Could you check a few things on this model? Use its own coordinates, in mm. A direction names the side the tool comes from. Coordinates: 2 decimals unless noted, no trailing zeros. Write each loop counter-clockwise with the first axis right and the second up, starting at its lowest first coordinate (ties: lowest second). Pieces come first, ordered by that corner, then holes. Notation, with made-up numbers: M 89.25,-30 L 123.25,-30 A7 ccw 123.25,-19 Z; hole C 46,-17.75 d2. An arc over 180 degrees is marked long. Answer as CSV lines item,"result". Start each with the question number.
Item 1: On a 3-axis mill with a long thin cutter (end or side, diameter ignored), from which of +Z, -Z, +X, -X, +Y, -Y can I reach the whole of each face in a straight line? I mean faces 4 (the cylindrical face through (-15.07, 3.24, 10.32)), 5 (the flat face through (15, 4.5, 4)), 6 (the flat face through (-15, -4.5, 4)), 7 (the flat face through (15, -4.5, 4)). Say none if no direction works.
Item 2: I'm going to push flat-ended pins straight in: P1, Ø3, axis at x = 14.5, z = 3.5, coming from the +Y side; P2, Ø1.5, axis at y = 6.5, z = 8.5, coming from the +X side; P3, Ø6.5, axis at x = 16, z = 4, coming from the -Y side; P4, Ø2.5, axis at y = 0, z = 6.6, coming from the +X side. Where does each tip first touch, or does it pass through?
Item 3: Suppose I cut it at C-C, the plane z = 4.25. Write out the boundary of the cut face in (x, y), and give its area (3 significant figures).
Item 4: Suppose I cut it at B-B, the plane x = -17. Write out the boundary of the cut face in (y, z).
Item 5: We'd pull the mould along Y, two halves only. Please class faces 1 (the cylindrical face through (9, -8, 7)), 2 (the cylindrical face through (-8, 9, 7)), 3 (the flat face through (0, 0, 1.2)): +Y half, -Y half, draft (parallel to the pull), parting line (faces both ways), or undercut.
Item 6: Suppose I cut it at D-D, the plane x = 0. Write out the boundary of the cut face in (y, z), and give its area (3 significant figures).
Item 7: If I drill on line 1 along Y through (x, z) = (-17, 6.6); line 2 along Y through (x, z) = (0, 9.5); line 3 along X through (y, z) = (5.5, 4.75), over which ranges is the centre line in solid material (lowest first)? Write a range as [from, to].
Item 8: Suppose I cut it at A-A, the plane z = 6.6. Write out the boundary of the cut face in (x, y).
```python
from build123d import *

# Parameters (mm, degrees)
F0_W        = 20
F0_H        = 20
F0_R        = 8.3
F1_DEPTH    = 15
F2_W        = 9
F2_H        = 12
F3_DEPTH    = 10
F4_W        = 9
F4_H        = 12
F4_R        = 1.6
F5_DEPTH    = 10
F6_DEPTH    = 30.001
F7_DEPTH    = 1.2
F8_T1_DEPTH = 40
F8_T3_DEPTH = 22.5
F8_T5_DEPTH = 22.5
F9_R        = 1


# Not quite as in the source:
# - a fillet or chamfer that OpenCascade refuses, or shapes differently, is made with other operations: its cross-section is extruded or revolved along the edge and cut away or added


with BuildPart() as f1:
    # F0 (on Top) → F1 (new body)
    with BuildSketch(Plane.XY):
        Rectangle(F0_W, F0_H)
        Circle(F0_R, mode=Mode.SUBTRACT)
    extrude(amount=F1_DEPTH)

    # F2 (on face) → F3 (join)
    with BuildSketch(Plane(origin=(-10, 0, 0), x_dir=(0, -1, 0), z_dir=(-1, 0, 0))):
        with Locations((0, 6)):
            Rectangle(F2_W, F2_H)
    extrude(amount=F3_DEPTH)

    # F4 (on face) → F5 (join)
    with BuildSketch(Plane.YZ.offset(10)):
        with Locations((0, 6)):
            Rectangle(F4_W, F4_H)
        with Locations((0, 6.6)):
            Circle(F4_R, mode=Mode.SUBTRACT)
    extrude(amount=F5_DEPTH)

    # F4 (on face) → F6 (cut, through all)
    with BuildSketch(Plane.YZ.offset(10)):
        with Locations((0, 6.6)):
            Circle(F4_R)
    extrude(amount=-F6_DEPTH, mode=Mode.SUBTRACT)

    # F0 (on Top) → F7 (join)
    with BuildSketch(Plane.XY):
        Circle(F0_R)
    extrude(amount=F7_DEPTH)

    # F8: fillet of radius 5 on 8 edges, made by hand

    # F8_s2 → F8_t1 (cut)
    with BuildSketch(Plane.XY.offset(-12.5)):
        with BuildLine():
            ThreePointArc((-10, -5), (-8.5355339059, -8.5355339059), (-5, -10))
            Line((-5, -10), (-10, -10))
            Line((-10, -10), (-10, -5))
        make_face()
        with BuildLine():
            ThreePointArc((10, -5), (8.5355339059, -8.5355339059), (5, -10))
            Line((5, -10), (10, -10))
            Line((10, -10), (10, -5))
        make_face()
        with BuildLine():
            ThreePointArc((-5, 10), (-8.5355339059, 8.5355339059), (-10, 5))
            Line((-10, 5), (-10, 10))
            Line((-10, 10), (-5, 10))
        make_face()
        with BuildLine():
            ThreePointArc((5, 10), (8.5355339059, 8.5355339059), (10, 5))
            Line((10, 5), (10, 10))
            Line((10, 10), (5, 10))
        make_face()
    extrude(amount=F8_T1_DEPTH, mode=Mode.SUBTRACT)

    # F8_s4 → F8_t3 (cut)
    with BuildSketch(Plane.YZ.offset(-32.5)):
        with BuildLine():
            ThreePointArc((4.5, 7), (3.0355339059, 10.5355339059), (-0.5, 12))
            Line((-0.5, 12), (4.5, 12))
            Line((4.5, 12), (4.5, 7))
        make_face()
        with BuildLine():
            ThreePointArc((0.5, 12), (-3.0355339059, 10.5355339059), (-4.5, 7))
            Line((-4.5, 7), (-4.5, 12))
            Line((-4.5, 12), (0.5, 12))
        make_face()
    extrude(amount=F8_T3_DEPTH, mode=Mode.SUBTRACT)

    # F8_s6 → F8_t5 (cut)
    with BuildSketch(Plane.YZ.offset(10)):
        with BuildLine():
            ThreePointArc((-0.5, 12), (3.0355339059, 10.5355339059), (4.5, 7))
            Line((4.5, 7), (4.5, 12))
            Line((4.5, 12), (-0.5, 12))
        make_face()
        with BuildLine():
            ThreePointArc((-4.5, 7), (-3.0355339059, 10.5355339059), (0.5, 12))
            Line((0.5, 12), (-4.5, 12))
            Line((-4.5, 12), (-4.5, 7))
        make_face()
    extrude(amount=F8_T5_DEPTH, mode=Mode.SUBTRACT)

    # F9
    f9_edges = [f1.edges().sort_by_distance(p)[0] for p in [
        (15, -4.5, 0),
        (15, 4.5, 0),
        (-15, 4.5, 0),
        (-15, -4.5, 0),
    ]]
    fillet(f9_edges, radius=F9_R)


solid = f1.part
```
Ans:
1,face 4,"+Z, -X, +Y"
1,face 5,"+Z, -Z, +X, +Y"
1,face 6,"+Z, -Z, -X, -Y"
1,face 7,"+Z, -Z, +X, -Y"
2,P1,"stops at y = 4.5"
2,P2,"stops at x = 9.94"
2,P3,"stops at y = -4.5"
2,P4,"passes through"
3,outline,"M -20,-4.5 L -10,-4.5 L -10,-5 A5 ccw -5,-10 L 5,-10 A5 ccw 10,-5 L 10,-4.5 L 20,-4.5 L 20,4.5 L 10,4.5 L 10,5 A5 ccw 5,10 L -5,10 A5 ccw -10,5 L -10,4.5 L -20,4.5 Z; hole C 0,0 d16.6"
3,area,"342 mm^2"
4,outline,"M -4.5,1 A1 ccw -3.5,0 L 3.5,0 A1 ccw 4.5,1 L 4.5,7 A5 ccw 0,11.97 A5 ccw -4.5,7 Z; hole C 0,6.6 d3.2"
5,face 1,"-Y half"
5,face 2,"+Y half"
5,face 3,"undercut"
6,outline,"M -10,0 L 10,0 L 10,15 L 8.3,15 L 8.3,1.2 L -8.3,1.2 L -8.3,15 L -10,15 Z"
6,area,"70.9 mm^2"
7,line 1,"y = [-4.5, -1.6], [1.6, 4.5]"
7,line 2,"y = [-10, -8.3], [8.3, 10]"
7,line 3,"x = [-9.97, -6.22], [6.22, 9.97]"
8,outline,"M -20,-4.5 L -10,-4.5 L -10,-5 A5 ccw -5,-10 L 5,-10 A5 ccw 10,-5 L 10,-4.5 L 20,-4.5 L 20,-1.6 L 8.14,-1.6 A8.3 cw -8.14,-1.6 L -20,-1.6 Z; M -20,1.6 L -8.14,1.6 A8.3 cw 8.14,1.6 L 20,1.6 L 20,4.5 L 10,4.5 L 10,5 A5 ccw 5,10 L -5,10 A5 ccw -10,5 L -10,4.5 L -20,4.5 Z"
